Geometry: final body of the model. Coordinates: model frame, mm. A direction names the side the tool comes from. Give positions to 0.01 mm unless a question says otherwise; leave off trailing zeros. Loops run counter-clockwise (first coordinate to the right, second up) from the corner with the lowest first, then second, coordinate; pieces in that order, holes last.
from build123d import *

# Parameters (mm, degrees)
SCHIZZO1_R                  = 30
ESTRUSIONE1_DEPTH           = 1136
SCHIZZO2_R                  = 27.5
ESTRUSIONE2_DEPTH           = 4
SCHIZZO3_R                  = 30
ESTRUSIONE3_DEPTH           = 35
SMUSSO1_SIZE                = 3
ESTRUSIONE4_START           = 4
SCHIZZO4_R                  = 27.5
ESTRUSIONE4_DEPTH           = 4
ESTRUSIONE5_START           = 35
SCHIZZO5_R                  = 30
ESTRUSIONE5_DEPTH           = 35
SMUSSO2_SIZE                = 3
ESTRUSIONE6_START           = -18
SCHIZZO6_R                  = 5
ESTRUSIONE6_DEPTH           = 1158.765707954
RIPETIZIONECIRCOLARE1_COUNT = 3


with BuildPart() as part:
    # Schizzo1 → Estrusione1 (new body)
    with BuildSketch(Plane(origin=(0, 0, 0), x_dir=(1, 0, 0), z_dir=(0, 1, 0))):
        with Locations(Location((0, 0, 0), (0, 0, 270))):
            Circle(SCHIZZO1_R)
    extrude(amount=ESTRUSIONE1_DEPTH)

    # Schizzo2 → Estrusione2 (add)
    with BuildSketch(Plane(origin=(0, 1136, 0), x_dir=(1, 0, 0), z_dir=(0, 1, 0))):
        with Locations(Location((0, 0, 0), (0, 0, 270))):
            Circle(SCHIZZO2_R)
    extrude(amount=ESTRUSIONE2_DEPTH)

    # Schizzo3 → Estrusione3 (add)
    with BuildSketch(Plane(origin=(0, 1140, 0), x_dir=(1, 0, 0), z_dir=(0, 1, 0))):
        with Locations(Location((0, 0, 0), (0, 0, 270))):
            Circle(SCHIZZO3_R)
    extrude(amount=ESTRUSIONE3_DEPTH)

    # Smusso1
    smusso1_edges = [part.edges().sort_by_distance(p)[0] for p in [
        (0, 1175, -30),
    ]]
    chamfer(smusso1_edges, length=SMUSSO1_SIZE)

    # Schizzo4 → Estrusione4 (add)
    with BuildSketch(Plane.XZ.offset(ESTRUSIONE4_START)):
        with Locations(Location((0, 0, 0), (0, 0, 90))):
            Circle(SCHIZZO4_R)
    extrude(amount=-ESTRUSIONE4_DEPTH)

    # Schizzo5 → Estrusione5 (add)
    with BuildSketch(Plane.XZ.offset(4).offset(ESTRUSIONE5_START)):
        with Locations(Location((0, 0, 0), (0, 0, 90))):
            Circle(SCHIZZO5_R)
    extrude(amount=-ESTRUSIONE5_DEPTH)

    # Smusso2
    smusso2_edges = [part.edges().sort_by_distance(p)[0] for p in [
        (0, -39, -30),
    ]]
    chamfer(smusso2_edges, length=SMUSSO2_SIZE)

    # Schizzo6 → Estrusione6 (cut, through all)
    with BuildSketch(Plane.XY.offset(ESTRUSIONE6_START)):
        with Locations((0, 704)):
            Circle(SCHIZZO6_R)
    estrusione6 = extrude(amount=-ESTRUSIONE6_DEPTH, mode=Mode.SUBTRACT)

    # RipetizioneCircolare1: Estrusione6 ×3 about axis
    ripetizionecircolare1_axis = Axis((0, 0, 0), (0, 1, 0))
    for i in range(1, RIPETIZIONECIRCOLARE1_COUNT):
        add(estrusione6.rotate(ripetizionecircolare1_axis, i * 360 / RIPETIZIONECIRCOLARE1_COUNT), mode=Mode.SUBTRACT)


solid = part.part
Item 1: Set-up query: faces 4 (the face through (0, -39, 0)), 5 (the face through (-24.3, 0, 13.2)). Return all of +Z, -Z, +X, -X, +Y, -Y with unobstructed straight access to the full face (end or side cutting, diameter ignored); none if empty.
Values follow:
face 4: +Z, -Z, +X, -X, -Y
face 5: none
Item 2: Section query A-A on y = 130. Return loops of the section in (x, z), plus the area to 3 significant figures.
Values follow:
outline: circle Ø60 at (0, 0)
area: 2,830 mm2
Item 3: Ray query, probe 1 along Y at (x, z) = (-11.5, 26); probe 2 along Y at (x, z) = (0, -24); probe 3 along X at (y, z) = (704, -27.25). Return the intervals inside material, ascending.
Values follow:
probe 1: y = -37.57 to -4, 0 to 1136, 1140 to 1173.57
probe 2: y = -39 to 699, 709 to 1175
probe 3: x = -12.55 to -5, 5 to 12.55
Item 4: Draft query along Y for faces 1 (the face through (26.5, -38.854, -5.885)), 2 (the face through (1.32, 1155.78, -29.97)), 3 (the face through (-24.397, 1137.972, 12.69)). Return one class per face: +Y half, -Y half, draft (parallel to the pull), parting line (faces both ways), or undercut.
Values follow:
face 1: -Y half
face 2: draft
face 3: undercut
Item 5: Pin query (flat end, axial travel): pin 1 (3 mm diameter, centred on x = 7, y = 693.5, fed in from +Z); pin 2 (9 mm diameter, centred on x = 0, y = 704, fed in from -Z); pin 3 (10 mm diameter, centred on x = -18, y = 733.5, fed in from +Z). Return the tip coordinate at first contact, or that it passes through.
Values follow:
pin 1: stops at z = 29.49
pin 2: stops at z = -18
pin 3: stops at z = 27.04
